Verification items for the finished model (mm, model axes). A direction names the side the tool comes from. Round coordinates to 2 decimals unless told otherwise and drop trailing zeros. Order: outer loops, then holes, each group sorted by start corner. A loop starts at its lowest first (then second) coordinate and runs counter-clockwise, first axis right, second up. Notation, with made-up numbers: M -3,-3.75 L 17,-3.75 A6 cw 17,6.25 Z; hole C 61,65 d10. An arc over 180 degrees is marked long. Use CSV: the item, a comma, the result in double quotes. Start each with the question number.
Q1. Gauge pin test, flat ends, axial feed: pin 1 Ø11.5 at (x, z) = (25.275, 11.25) entering from -Y; pin 2 Ø8 at (y, z) = (25.275, 11.25) entering from +X; pin 3 Ø5 at (x, z) = (19, 10) entering from +Y. Record the tip position at first contact, or that the pin passes through.
Q2. Scan lines: line 1 (Y direction, x = 0.85, z = 11.25); line 2 (X direction, y = 22.5, z = 5.5). Record each from-to range of solid material in increasing order.
Q3. Sectioned sample at D-D (x = 6.5). Enter the section's corners in (y, z).
Q4. Sectioned sample at C-C (z = 3.5). Enter the section's corners in (x, y).
Q5. Mould release check, pull along Z, two halves, no side actions. Record for faces 1 (the face through (22, 4, 9)), 2 (the face through (25.12, 2.03, 14.82)), 3 (the face through (11, 3.8, 22.5)), 4 (the face through (11, 3.8, 0)): +Z half, -Z half, draft (parallel to the pull), parting line (faces both ways), or undercut.
Q6. Set-up check for faces 5 (the face through (2.028, 28.765, 10.475)), 6 (the face through (4, 22, 9)): record each of +Z, -Z, +X, -X, +Y, -Y from which the full face is reachable in a straight line by a thin tool's end or side.
Q7. Sectioned sample at B-B (y = 3.5). Enter the section's corners in (x, z) (3 decimals).
Q8. Sectioned sample at A-A (z = 11.25). Enter the section's corners in (x, y).
Autodesk Inventor part; units mm, degrees
ref_plane "YZ Plane" through (0, 0, 0) normal (1, 0, 0) x (0, 1, 0)
ref_plane "XZ Plane" through (0, 0, 0) normal (0, 1, 0) x (-1, 0, 0)
ref_plane "XY Plane" through (0, 0, 0) normal (0, 0, 1) x (1, 0, 0)
sketch "Sketch2" plane through (0, 0, 0) normal (0, 0, 1) x (1, 0, 0)
  line L0 (0, 0) -> (40, 0)
  line L1 (40, 0) -> (40, 4)
  line L2 (40, 4) -> (0, 4)
  line L3 (0, 4) -> (0, 0)
  line L4 (0, 0) -> (4, 0)
  line L5 (4, 0) -> (4, 40)
  line L6 (4, 40) -> (0, 40)
  line L7 (0, 40) -> (0, 0)
  point P0 (4, 4)
  point P1 (0, 4)
  dimension "d0" = 40
  dimension "d1" = 40
  dimension "d2" = 4
  dimension "d3" = 4
extrude "Extrusion1" add sketch "Sketch2" along normal blind 22.5
sketch "Sketch3" plane through (0, 0, 0) normal (0, -1, 0) x (1, 0, 0)
  circle A0 centre (25.275, 11.25) radius 5.756
  line L0 (0, 22.5) -> (40, 22.5)
  line L1 (0, 0) -> (0, 22.5)
  dimension "d6" = 11.25
  dimension "d7" = 25.275
sketch "Sketch4" plane through (0, 0, 0) normal (-1, 0, 0) x (0, 0, 1)
  circle A0 centre (11.25, 25.275) radius 7.6084
  line L0 (22.5, 40) -> (22.5, 0)
  line L1 (0, 0) -> (22.5, 0)
  line L2 (0, 40) -> (22.5, 40)
  dimension "d8" = 11.25
  dimension "d9" = 25.275
  dimension "d24" = 14.725
hole "Hole1" at (0, 25.275, 11.25) direction (1, 0, 0) diameter 7.15 depth 5
hole "Hole2" at (25.275, 0, 11.25) direction (0, 1, 0) diameter 7.15 depth 5
properties part number "Lbracket"
Verdict:
1,pin 1,"stops at y = 0"
1,pin 2,"stops at x = 4"
1,pin 3,"stops at y = 4"
2,line 1,"y = 0 to 21.7, 28.85 to 40"
2,line 2,"x = 0 to 4"
3,outline,"M 0,0 L 4,0 L 4,22.5 L 0,22.5 Z"
4,outline,"M 0,0 L 40,0 L 40,4 L 4,4 L 4,40 L 0,40 Z"
5,face 1,"draft"
5,face 2,"undercut"
5,face 3,"+Z half"
5,face 4,"-Z half"
6,face 5,"+X, -X"
6,face 6,"+Z, -Z, +X, +Y"
7,outline,"M 0,0 L 40,0 L 40,22.5 L 0,22.5 Z; hole C 25.275,11.25 d7.15"
8,outline,"M 0,0 L 21.7,0 L 21.7,4 L 4,4 L 4,21.7 L 0,21.7 Z; M 0,28.85 L 4,28.85 L 4,40 L 0,40 Z; M 28.85,0 L 40,0 L 40,4 L 28.85,4 Z"
